Geometry check sheet. Reference: the model listing, model coordinates, mm. A direction names the side the tool comes from. Round coordinates to 2 decimals unless told otherwise and drop trailing zeros. Order: outer loops, then holes, each group sorted by start corner. A loop starts at its lowest first (then second) coordinate and runs counter-clockwise, first axis right, second up.
(1) Cross-section at B-B on z = 0. Count the separate pieces of the cut face and the enclosed holes in it, and give its area (3 significant figures).
(2) Set-up check for faces 1 (the face through (2.48, 10.46, -0.33)), 2 (the face through (10.845, 4.799, -3.582)), 3 (the face through (-7.88, 1.27, 1.27)), 4 (the face through (-1.74, 2.81, -0.03)): record each of +Z, -Z, +X, -X, +Y, -Y from which the full face is reachable in a straight line by a thin tool's end or side.
(3) Gauge pin test, flat ends, axial feed: P1, Ø1.8, axis at x = 7, y = 7, coming from the -Z side; P2, Ø2, axis at x = -6.5, z = 2.5, coming from the +Y side (3 decimals); P3, Ø3.5, axis at x = 7.94, y = 5.72, coming from the -Z side; P4, Ø5.5, axis at x = 0, y = 5.715, coming from the +Z side. Record the tip position at first contact, or that the pin passes through.
(4) Cross-section at A-A on x = 0. Enter the section's corners in (y, z) (3 decimals), and give its area (3 significant figures).
(5) Cross-section at D-D on x = -10. Enter the section's corners in (y, z) (3 decimals).
(6) Draft check along X on faces 5 (the face through (-0.2, 2.5, 3.969)), 6 (the face through (11.19, 8.72, -0.46)). Enter one of: pulls with the +X half, pulls with the -X half, needs draft (parallel to the pull), parting line crosses it, or undercut.
(7) Thickness scan on L1, parallel to X at y = 8.9, z = 0 (3 decimals); L2, parallel to Y at x = 0, z = 3.2 (3 decimals); L3, parallel to Z at x = 14, y = 1.25. Record the ranges inside material, lowest first.
from build123d import *

# Parameters (mm, degrees)
SKETCH1_W                = 31.75
SKETCH1_H                = 7.9375
BASE_EXTRUDE_DEPTH       = 9.525
SKETCH2_R                = 2.4384
BOSS_EXTRUDE1_DEPTH      = 1.905
LPATTERN4_COUNT          = 4
LPATTERN4_PITCH          = 7.9375
SHELL1_T                 = -1.5875
SKETCH5_R                = 2.3876
CUT_EXTRUDE1_DEPTH       = 22.110765767
SKETCH6_R                = 3.048
CBORE1_DEPTH             = 0.508
CBORE2_START             = -0.762
SKETCH7_R                = 3.048
CBORE2_DEPTH             = 0.762
BOSS_EXTRUDE_THIN1_START = -5.842
SKETCH8_R                = 3.3876
SKETCH8_R_2              = 2.3876
BOSS_EXTRUDE_THIN1_DEPTH = 4.7625
LPATTERN7_COUNT          = 3
LPATTERN7_PITCH          = 7.9375
INSDOT2_REACH            = 21.96
INSDOT2_END_RADIUS       = 3.3876
SKETCH4_R                = 1.27
LPATTERN6_COUNT          = 3
LPATTERN6_PITCH          = 7.9375
CUT_EXTRUDE2_START       = -1.905
SKETCH10_R               = 1.524
CUT_EXTRUDE2_DEPTH       = 1.905
LPATTERN8_COUNT          = 4
LPATTERN8_PITCH          = 7.9375
FILLET1_R                = 0.254


with BuildPart() as part:
    # Sketch1 → Base-Extrude (new body)
    with BuildSketch(Plane(origin=(0, 0, 0), x_dir=(1, 0, 0), z_dir=(0, 1, 0))):
        Rectangle(SKETCH1_W, SKETCH1_H)
    extrude(amount=BASE_EXTRUDE_DEPTH)

    # Sketch2 → Boss-Extrude1 (add)
    with BuildSketch(Plane(origin=(0, 9.525, 0), x_dir=(-1, 0, 0), z_dir=(0, 1, 0))):
        with Locations(Location((11.90625, 0, 0), (0, 0, 270))):
            Circle(SKETCH2_R)
    boss_extrude1 = extrude(amount=BOSS_EXTRUDE1_DEPTH)

    # LPattern4: Boss-Extrude1 ×4
    with Locations(*[(i * LPATTERN4_PITCH, 0, 0) for i in range(1, LPATTERN4_COUNT)]):
        add(boss_extrude1)

    # Shell1
    shell1_openings = [part.faces().sort_by_distance(p)[0] for p in [
        (0, 0, 0),
    ]]
    offset(amount=SHELL1_T, openings=shell1_openings, kind=Kind.INTERSECTION)

    # Sketch5 → Cut-Extrude1 (cut, through all)
    with BuildSketch(Plane.XY.offset(3.96875)):
        with Locations((-7.9375, 5.715)):
            Circle(SKETCH5_R)
    cut_extrude1 = extrude(amount=-CUT_EXTRUDE1_DEPTH, mode=Mode.SUBTRACT)

    # Sketch6 → cbore1 (cut)
    with BuildSketch(Plane.XY.offset(3.96875)):
        with Locations((-7.9375, 5.715)):
            Circle(SKETCH6_R)
    cbore1 = extrude(amount=-CBORE1_DEPTH, mode=Mode.SUBTRACT)

    # Sketch7 → cbore2 (cut)
    with BuildSketch(Plane(origin=(0, 0, -3.96875), x_dir=(-1, 0, 0), z_dir=(0, 0, -1)).offset(CBORE2_START)):
        with Locations(Location((7.9375, 5.715, 0), (0, 0, 180))):
            Circle(SKETCH7_R)
    cbore2 = extrude(amount=CBORE2_DEPTH, mode=Mode.SUBTRACT)

    # Sketch8 → Boss-Extrude-Thin1 (add)
    with BuildSketch(Plane.XY.offset(3.46075).offset(BOSS_EXTRUDE_THIN1_START)):
        with Locations((-7.9375, 5.715)):
            Circle(SKETCH8_R)
        with Locations((-7.9375, 5.715)):
            Circle(SKETCH8_R_2, mode=Mode.SUBTRACT)
    boss_extrude_thin1 = extrude(amount=BOSS_EXTRUDE_THIN1_DEPTH)

    # LPattern7: Cut-Extrude1, cbore1, cbore2, Boss-Extrude-Thin1 ×3
    with Locations(*[(i * LPATTERN7_PITCH, 0, 0) for i in range(1, LPATTERN7_COUNT)]):
        add(cut_extrude1, mode=Mode.SUBTRACT)
        add(cbore1, mode=Mode.SUBTRACT)
        add(cbore2, mode=Mode.SUBTRACT)
        add(boss_extrude_thin1)

    # InsDot2: up to this cylinder (the profile starts outside it)
    insdot2_end = Plane(origin=(7.9375, 5.715, 0), z_dir=(0, 0, 1)) * Cylinder(INSDOT2_END_RADIUS, 51.6952, mode=Mode.PRIVATE)
    # Sketch4 → InsDot2 (add, up to the surface)
    with BuildSketch(Plane.XZ, mode=Mode.PRIVATE) as insdot2_sk1:
        with Locations(Location((7.9375, 0, 0), (0, 0, 270))):
            Circle(SKETCH4_R)
    insdot2_tool1 = extrude(insdot2_sk1.sketch, amount=-INSDOT2_REACH, mode=Mode.PRIVATE) - insdot2_end
    insdot2 = insdot2_tool1.solids().sort_by_distance((7.9375, 0, 0))[0]
    add(insdot2)

    # LPattern6: InsDot2 ×3
    with Locations(*[(-i * LPATTERN6_PITCH, 0, 0) for i in range(1, LPATTERN6_COUNT)]):
        add(insdot2)

    # Sketch10 → Cut-Extrude2 (cut)
    with BuildSketch(Plane(origin=(0, 11.43, 0), x_dir=(-1, 0, 0), z_dir=(0, 1, 0)).offset(CUT_EXTRUDE2_START)):
        with Locations(Location((11.90625, 0, 0), (0, 0, 90))):
            Circle(SKETCH10_R)
    cut_extrude2 = extrude(amount=CUT_EXTRUDE2_DEPTH, mode=Mode.SUBTRACT)

    # LPattern8: Cut-Extrude2 ×4
    with Locations(*[(i * LPATTERN8_PITCH, 0, 0) for i in range(1, LPATTERN8_COUNT)]):
        add(cut_extrude2, mode=Mode.SUBTRACT)

    # Fillet1
    fillet1_edges = [part.edges().sort_by_distance(p)[0] for p in [
        (15.875, 9.525, 0),
        (0, 9.525, -3.96875),
        (-15.875, 9.525, 0),
        (0, 9.525, 3.96875),
    ]]
    fillet(fillet1_edges, radius=FILLET1_R)


solid = part.part
Found:
1. separate pieces: 5
1. enclosed holes: 3
1. area: 139 mm2
2. face 1: +Y
2. face 2: -Z
2. face 3: -Y
2. face 4: none
3. P1: stops at z = -3.21
3. P2: stops at y = 9.525
3. P3: passes through
3. P4: stops at z = 3.46
4. outline: (0, -3.969) - (2.667, -3.969) - (2.667, -3.207) - (3.327, -3.207) - (3.327, 3.461) - (2.667, 3.461) - (2.667, 3.969) - (0, 3.969) - (0, 2.381) - (2.327, 2.381) - (2.327, 1.27) - (0, 1.27) - (0, -1.27) - (2.327, -1.27) - (2.327, -2.381) - (0, -2.381) - close; (8.103, -3.207) - (8.763, -3.207) - (8.763, -3.969) - (9.271, -3.969) arc R0.254 ccw to (9.525, -3.715) - (9.525, 3.715) arc R0.254 ccw to (9.271, 3.969) - (8.763, 3.969) - (8.763, 3.461) - (8.103, 3.461) - close
4. area: 30.8 mm2
5. outline: (0, -3.969) - (3.471, -3.969) - (3.471, -3.207) - (4.512, -3.207) - (4.512, 3.461) - (3.471, 3.461) - (3.471, 3.969) - (0, 3.969) - (0, 2.381) - (3.028, 2.381) - (3.028, -2.381) - (0, -2.381) - close; (6.918, -3.207) - (7.959, -3.207) - (7.959, -3.969) - (9.271, -3.969) arc R0.254 ccw to (9.525, -3.715) - (9.525, -1.521) - (11.43, -1.521) - (11.43, 1.521) - (9.525, 1.521) - (9.525, 3.715) arc R0.254 ccw to (9.271, 3.969) - (7.959, 3.969) - (7.959, 3.461) - (6.918, 3.461) - close
6. face 5: needs draft
6. face 6: undercut
7. L1: x = -15.875 to -12.757, -11.055 to -4.82, -3.118 to 3.118, 4.82 to 11.055, 12.757 to 15.875
7. L2: y = 0 to 3.327, 8.103 to 9.525
7. L3: z = -3.97 to -2.38, 2.38 to 3.97
